```python
from build123d import *

# Parameters (mm, degrees)
SKETCH1_W           = 6.35
SKETCH1_H           = 12.7
BOSS_EXTRUDE1_DEPTH = 3.175
CUT_EXTRUDE1_DEPTH  = 7.35


with BuildPart() as part:
    # Sketch1 → Boss-Extrude1 (new body, symmetric)
    with BuildSketch(Plane.XY):
        Polygon((-50.8, -9.525), (50.8, -9.525), (50.8, -6.35), (57.15, -6.35), (57.15, 6.35), (50.8, 6.35), (50.8, 9.525), (-50.8, 9.525), (-50.8, 6.35), (-57.15, 6.35), (-57.15, -6.35), (-50.8, -6.35), align=None)
        with Locations((-22.675, 0)):
            Rectangle(SKETCH1_W, SKETCH1_H, mode=Mode.SUBTRACT)
        with Locations((22.675, 0)):
            Rectangle(SKETCH1_W, SKETCH1_H, mode=Mode.SUBTRACT)
    extrude(amount=BOSS_EXTRUDE1_DEPTH, both=True)

    # Sketch2 → Cut-Extrude1 (cut, through all)
    with BuildSketch(Plane.XY.offset(3.175)):
        Polygon((-31.840276407, 6.35), (-47.625, 6.35), (-47.625, -4.427741378), align=None)
        Polygon((-29.025, 4.427741378), (-44.809723593, -6.35), (-29.025, -6.35), align=None)
        Polygon((-16.325, -4.646633401), (-4.379127517, 0), (-16.325, 4.646633401), align=None)
        Polygon((-11.945872483, 6.35), (0, 1.703366599), (11.945872483, 6.35), align=None)
        Polygon((4.379127517, 0), (16.325, -4.646633401), (16.325, 4.646633401), align=None)
        Polygon((-11.945872483, -6.35), (11.945872483, -6.35), (0, -1.703366599), align=None)
        Polygon((44.809723593, -6.35), (29.025, 4.427741378), (29.025, -6.35), align=None)
        Polygon((47.625, 6.35), (31.840276407, 6.35), (47.625, -4.427741378), align=None)
    extrude(amount=-CUT_EXTRUDE1_DEPTH, mode=Mode.SUBTRACT)


solid = part.part
```
Source: CAD feature listing. Evaluate the final solid. Frame: model axes, mm. A direction names the side the tool comes from. Coordinates: 2 decimals unless noted, no trailing zeros. Write each loop counter-clockwise with the first axis right and the second up, starting at its lowest first coordinate (ties: lowest second). Pieces come first, ordered by that corner, then holes. Notation, with made-up numbers: (58.5, -39) -> (113.5, -39) arc R3 ccw to (113.5, -35) -> close; hole circle Ø4 at (74, -22.5). An arc over 180 degrees is marked (long way). Return JSON: item names as keys, results as strings. Group by question number.
1) Set-up query: faces 5 (the face through (-54, 6.35, 0)), 6 (the face through (-36.81, -0.89, 0.04)), 7 (the face through (54, 6.35, 0)), 8 (the face through (50.8, -8, 0)). Return all of +Z, -Z, +X, -X, +Y, -Y with unobstructed straight access to the full face (end or side cutting, diameter ignored); none if empty.
2) Section query A-A, the plane x = -14. Return loops of the section in (y, z) (3 decimals).
3) Section query D-D, the plane x = -33. Return loops of the section in (y, z) (3 decimals), plus the area to 3 significant figures.
4) Ray query, line 1 along Y through (x, z) = (23.5, -2) (3 decimals); line 2 along Y through (x, z) = (10.5, -2.25) (3 decimals); line 3 along Y through (x, z) = (33, -2.5) (3 decimals). Return the intervals inside material, ascending.
5) Mould query, pull axis X, two halves, no side actions, for faces 1 (the face through (-19.5, 0, 0)), 2 (the face through (57.15, 0, 0)), 3 (the face through (-1, 0, 3.175)), 4 (the face through (-16.325, 0, 0)). Classes: +X half, -X half, draft (parallel to the pull), parting line (faces both ways), or undercut.
6) Contact query for flat-ended pins moving along their axis: P1, Ø1.6, axis at y = 7.5, z = 0, coming from the -X side; P2, Ø1.9, axis at x = -53, z = 0, coming from the +Y side; P3, Ø3, axis at x = -53, z = 0, coming from the -Y side. Output: stop coordinate, or through.
7) Section query C-C, the plane z = 1.75. State how many separate pieces and enclosed holes the cut face has, plus the area to 3 significant figures.
8) Section query B-B, the plane x = 9.5. Return loops of the section in (y, z) (3 decimals).
From the geometry:
{
 "1": {"face 5": "+Z, -Z, -X, +Y", "face 6": "+Z, -Z", "face 7": "+Z, -Z, +X, +Y", "face 8": "+Z, -Z, +X, -Y"},
 "2": {"outline": "(-9.525, -3.175) -> (-3.742, -3.175) -> (-3.742, 3.175) -> (-9.525, 3.175) -> close; (3.742, -3.175) -> (9.525, -3.175) -> (9.525, 3.175) -> (3.742, 3.175) -> close"},
 "3": {"outline": "(-9.525, -3.175) -> (-6.35, -3.175) -> (-6.35, 3.175) -> (-9.525, 3.175) -> close; (1.714, -3.175) -> (5.558, -3.175) -> (5.558, 3.175) -> (1.714, 3.175) -> close; (6.35, -3.175) -> (9.525, -3.175) -> (9.525, 3.175) -> (6.35, 3.175) -> close", "area": "64.7 mm²"},
 "4": {"line 1": "-9.525 to -6.35, 6.35 to 9.525", "line 2": "-9.525 to -6.35, -5.788 to -2.381, 2.381 to 5.788, 6.35 to 9.525", "line 3": "-9.525 to -6.35, 1.714 to 5.558, 6.35 to 9.525"},
 "5": {"face 1": "undercut", "face 2": "+X half", "face 3": "draft", "face 4": "undercut"},
 "6": {"P1": "x = -50.8", "P2": "y = 6.35", "P3": "y = -6.35"},
 "7": {"separate pieces": "1", "enclosed holes": "10", "area": "1,370 mm²"},
 "8": {"outline": "(-9.525, -3.175) -> (-6.35, -3.175) -> (-6.35, 3.175) -> (-9.525, 3.175) -> close; (-5.399, -3.175) -> (-1.992, -3.175) -> (-1.992, 3.175) -> (-5.399, 3.175) -> close; (1.992, -3.175) -> (5.399, -3.175) -> (5.399, 3.175) -> (1.992, 3.175) -> close; (6.35, -3.175) -> (9.525, -3.175) -> (9.525, 3.175) -> (6.35, 3.175) -> close"}
}
